```python
from build123d import *

# Parameters (mm, degrees)
SKETCH1_W                = 82.55
SKETCH1_H                = 53.594
BOSS_EXTRUDE1_DEPTH      = 5.334
CUT_EXTRUDE1_START       = -88.085249325
CUT_EXTRUDE1_OUTLINE_W   = 5.334
CUT_EXTRUDE1_OUTLINE_H   = 5.334
CUT_EXTRUDE1_DEPTH       = 16.51
CUT_EXTRUDE1_START_2     = -55.065249325
CUT_EXTRUDE1_2_OUTLINE_W = 5.334
CUT_EXTRUDE1_2_OUTLINE_H = 5.334
CUT_EXTRUDE1_2_DEPTH     = 16.51
CUT_EXTRUDE1_START_3     = -22.045249325
CUT_EXTRUDE1_3_OUTLINE_W = 5.334
CUT_EXTRUDE1_3_OUTLINE_H = 5.334
CUT_EXTRUDE1_3_DEPTH     = 16.51
SKETCH3_W                = 5.334
SKETCH3_H                = 12.154056038
CUT_EXTRUDE2_DEPTH       = 97.676684204
SKETCH4_R                = 3.556
SKETCH4_R_2              = 1.524
CUT_EXTRUDE3_DEPTH       = 97.676684204


# Read off the part's stored shape, not the designer's step: Cut-Extrude1
with BuildPart() as part:
    # Sketch1 → Boss-Extrude1 (new body)
    with BuildSketch(Plane.XY):
        with Locations((-46.810249325, -12.686142782)):
            Rectangle(SKETCH1_W, SKETCH1_H)
    extrude(amount=BOSS_EXTRUDE1_DEPTH)

    # Cut-Extrude1 outline → Cut-Extrude1 (cut)
    with BuildSketch(Plane.YZ.offset(CUT_EXTRUDE1_START)):
        with Locations((11.443857218, 2.667)):
            Rectangle(CUT_EXTRUDE1_OUTLINE_W, CUT_EXTRUDE1_OUTLINE_H)
    extrude(amount=CUT_EXTRUDE1_DEPTH, mode=Mode.SUBTRACT)

    # Cut-Extrude1 2 outline → Cut-Extrude1 2 (cut)
    with BuildSketch(Plane.YZ.offset(CUT_EXTRUDE1_START_2)):
        with Locations((11.443857218, 2.667)):
            Rectangle(CUT_EXTRUDE1_2_OUTLINE_W, CUT_EXTRUDE1_2_OUTLINE_H)
    extrude(amount=CUT_EXTRUDE1_2_DEPTH, mode=Mode.SUBTRACT)

    # Cut-Extrude1 3 outline → Cut-Extrude1 3 (cut)
    with BuildSketch(Plane.YZ.offset(CUT_EXTRUDE1_START_3)):
        with Locations((11.443857218, 2.667)):
            Rectangle(CUT_EXTRUDE1_3_OUTLINE_W, CUT_EXTRUDE1_3_OUTLINE_H)
    extrude(amount=CUT_EXTRUDE1_3_DEPTH, mode=Mode.SUBTRACT)

    # Sketch3 → Cut-Extrude2 (cut, through all)
    with BuildSketch(Plane.XY.offset(5.334)):
        with Locations((-85.418249325, -33.406114763)):
            Rectangle(SKETCH3_W, SKETCH3_H)
        with Locations((-85.418249325, -9.098002686)):
            Rectangle(SKETCH3_W, SKETCH3_H)
        with Locations((-8.202249325, -33.406114763)):
            Rectangle(SKETCH3_W, SKETCH3_H)
        with Locations((-8.202249325, -9.098002686)):
            Rectangle(SKETCH3_W, SKETCH3_H)
    extrude(amount=-CUT_EXTRUDE2_DEPTH, mode=Mode.SUBTRACT)

    # Sketch4 → Cut-Extrude3 (cut, through all)
    with BuildSketch(Plane.XY.offset(5.334)):
        with Locations((-46.810249325, -15.353142782)):
            Circle(SKETCH4_R)
        with Locations((-55.331949325, -15.353142782)):
            Circle(SKETCH4_R_2)
        with Locations(Location((-38.288549325, -15.353142782, 0), (0, 0, 180))):
            Circle(SKETCH4_R_2)
    extrude(amount=-CUT_EXTRUDE3_DEPTH, mode=Mode.SUBTRACT)


solid = part.part
```
Model file for the job. Use its own axes, mm. A direction names the side the tool comes from. Give positions to 0.01 mm unless a question says otherwise; leave off trailing zeros. Write each loop counter-clockwise with the first axis right and the second up, starting at its lowest first coordinate (ties: lowest second). Pieces come first, ordered by that corner, then holes. Notation, with made-up numbers: M 24.5,-25.75 L 62.5,-25.75 A14 cw 62.5,-6.75 Z; hole C 5,66.5 d10. An arc over 180 degrees is marked long. Use a Markdown table: item, result.
1) Drill centre lines: line 1 (X direction, y = 9, z = 1.4); line 2 (X direction, y = -4.5, z = 4.45); line 3 (Y direction, x = -38.5, z = 2.2). Where is each one in solid material? Low to high. Write a range as from..to.
Responses:
| item | result |
|---|---|
| line 1 | x = -71.58..-55.07, -38.56..-22.05 |
| line 2 | x = -82.75..-10.87 |
| line 3 | y = -39.48..-16.86, -13.84..14.11 |
2) Pull direction X, two halves, no side cores. Call faces 1 (the flat face through (-38.555, 11, 3)), 2 (the flat face through (-10.869, -33, 3)), 3 (the flat face through (-30, 14.111, 3)), 4 (the flat face through (-55.065, 11, 3)): +X half, -X half, draft (parallel to the pull), parting line (faces both ways), or undercut.
Responses:
| item | result |
|---|---|
| face 1 | undercut |
| face 2 | +X half |
| face 3 | draft |
| face 4 | undercut |
3) Tool access for faces 5 (the flat face through (-8, -27.329, 3)), 6 (the flat face through (-85, -27.329, 3)), 7 (the flat face through (-71.575, 11, 3)), 8 (the flat face through (-14, 8.777, 3)): list every direction of +Z, -Z, +X, -X, +Y, -Y with a clear straight run to the whole face (end or side of a thin tool).
Responses:
| item | result |
|---|---|
| face 5 | +Z, -Z, +X, -Y |
| face 6 | +Z, -Z, -X, -Y |
| face 7 | +Z, -Z, -X, +Y |
| face 8 | +Z, -Z, +X, +Y |
4) Cut at C-C (y = -36). List the corners of the cut face in (x, z).
Responses:
| item | result |
|---|---|
| outline | M -82.75,0 L -10.87,0 L -10.87,5.33 L -82.75,5.33 Z |
5) Cut at A-A (y = -18). List the corners of the cut face in (x, z), and give its area (3 significant figures).
Responses:
| item | result |
|---|---|
| outline | M -88.09,0 L -49.18,0 L -49.18,5.33 L -88.09,5.33 Z; M -44.44,0 L -5.54,0 L -5.54,5.33 L -44.44,5.33 Z |
| area | 415 mm2 |
6) Cut at B-B (z = 3.35). List the corners of the cut face in (x, y), and give its area (3 significant figures).
Responses:
| item | result |
|---|---|
| outline | M -88.09,-27.33 L -82.75,-27.33 L -82.75,-39.48 L -10.87,-39.48 L -10.87,-27.33 L -5.54,-27.33 L -5.54,-15.18 L -10.87,-15.18 L -10.87,-3.02 L -5.54,-3.02 L -5.54,8.78 L -22.05,8.78 L -22.05,14.11 L -38.56,14.11 L -38.56,8.78 L -55.07,8.78 L -55.07,14.11 L -71.58,14.11 L -71.58,8.78 L -88.09,8.78 L -88.09,-3.02 L -82.75,-3.02 L -82.75,-15.18 L -88.09,-15.18 Z; hole C -55.33,-15.35 d3.05; hole C -46.81,-15.35 d7.11; hole C -38.29,-15.35 d3.05 |
| area | 3,850 mm2 |
7) Pin check, flat tips, straight feed: pin 1 (2.5 mm diameter, centred on y = -31, z = 3, fed in from -X); pin 2 (1.5 mm diameter, centred on x = -45, z = 2.5, fed in from +Y); pin 3 (2.5 mm diameter, centred on y = 12.5, z = 3.5, fed in from -X). Stop position of each tip, or through.
Responses:
| item | result |
|---|---|
| pin 1 | stops at x = -82.75 |
| pin 2 | stops at y = 8.78 |
| pin 3 | stops at x = -71.58 |
